```python
from build123d import *

# Parameters (mm, degrees)
SKETCH2_R          = 17.5
SKETCH2_R_2        = 6.5
PLATE_DEPTH        = 1
SKETCH2_4_R        = 3.5
ROD_DEPTH          = 125
SKETCH3_R          = 2.5
CUT_EXTRUDE1_DEPTH = 127


with BuildPart() as part:
    # Sketch2 → Plate (new body, symmetric)
    with BuildSketch(Plane(origin=(0, 0, 0), x_dir=(1, 0, 0), z_dir=(0, 1, 0))):
        Circle(SKETCH2_R)
        Circle(SKETCH2_R_2, mode=Mode.SUBTRACT)
    extrude(amount=PLATE_DEPTH, both=True)

    # Sketch2<4> → Rod (add)
    with BuildSketch(Plane(origin=(0, 0, 0), x_dir=(1, 0, 0), z_dir=(0, 1, 0))):
        with Locations((0, -12)):
            Circle(SKETCH2_4_R)
    extrude(amount=ROD_DEPTH)

    # Sketch3 → Cut-Extrude1 (cut, through all)
    with BuildSketch(Plane(origin=(0, 125, 0), x_dir=(1, 0, 0), z_dir=(0, 1, 0))):
        with Locations((0, -12)):
            Circle(SKETCH3_R)
    extrude(amount=-CUT_EXTRUDE1_DEPTH, mode=Mode.SUBTRACT)


solid = part.part
```
Model file for the job. Use its own axes, mm. Coordinates: 2 decimals unless noted, no trailing zeros. Write each loop counter-clockwise with the first axis right and the second up, starting at its lowest first coordinate (ties: lowest second). Pieces come first, ordered by that corner, then holes. Notation, with made-up numbers: (-22.75, 67) - (-6.75, 67) arc R23 ccw to (-6.75, 78) - close; hole circle Ø11 at (-31, -17.5). An arc over 180 degrees is marked (long way). One line per item, written item: value. Start each with the question number.
1. Mould opens along X. For faces 1 (the cylindrical face through (-5.158, -0.014, 3.955)), 2 (the flat face through (2, 125, 14)), 3 (the cylindrical face through (-0.759, 62.132, 15.417)) say: released by +X, released by -X, zero draft, split by the parting line, or undercut.
2. Probe line 1 (Z direction, x = 0, y = 0); line 2 (X direction, y = 98, z = 12); line 3 (X direction, y = 0, z = 0). List the from-to ranges inside material, lowest first. Write a range as from..to.
3. Slice it at A-A (z = 0). Write the cut outline in (x, y), plus the area to 3 significant figures.
4. Slice it at D-D (x = -10.5). Write the cut outline in (y, z), plus the area to 3 significant figures.
5. Slice it at C-C (y = 8). Write the cut outline in (x, z).
6. Slice it at B-B (x = 0). Write the cut outline in (y, z), plus the area to 3 significant figures.
7. Flat gauge pin, fed straight in: pin 1 (2 mm diameter, centred on x = 6.5, z = -9, fed in from +Y). Where does the tip first touch, or does it go through?
Answers below:
1. face 1: undercut
1. face 2: zero draft
1. face 3: split by the parting line
2. line 1: z = -17.5..-6.5, 6.5..9.5, 14.5..17.5
2. line 2: x = -3.5..-2.5, 2.5..3.5
2. line 3: x = -17.5..-6.5, 6.5..17.5
3. outline: (-17.5, -1) - (-6.5, -1) - (-6.5, 1) - (-17.5, 1) - close; (6.5, -1) - (17.5, -1) - (17.5, 1) - (6.5, 1) - close
3. area: 44.0 mm^2
4. outline: (-1, -14) - (1, -14) - (1, 14) - (-1, 14) - close
4. area: 56.0 mm^2
5. outline: circle Ø7 at (0, 12); hole circle Ø5 at (0, 12)
6. outline: (-1, -17.5) - (1, -17.5) - (1, -6.5) - (-1, -6.5) - close; (-1, 6.5) - (1, 6.5) - (1, 8.5) - (125, 8.5) - (125, 9.5) - (-1, 9.5) - close; (-1, 14.5) - (125, 14.5) - (125, 15.5) - (1, 15.5) - (1, 17.5) - (-1, 17.5) - close
6. area: 282 mm^2
7. pin 1: stops at y = 1
